Source: CAD feature listing. Evaluate the final solid. Frame: model axes, mm. Give positions to 0.01 mm unless a question says otherwise; leave off trailing zeros. Order: outer loops, then holes, each group sorted by start corner. A loop starts at its lowest first (then second) coordinate and runs counter-clockwise, first axis right, second up. Notation, with made-up numbers: M 81.5,69.25 L 93.5,69.25 A23 ccw 93.5,87.25 Z; hole C 80.25,47 d1. An arc over 180 degrees is marked long. Return JSON: item names as keys, results as strings.
Autodesk Inventor part; units mm, degrees
ref_plane "YZ Plane" through (0, 0, 0) normal (1, 0, 0) x (0, 1, 0)
ref_plane "XZ Plane" through (0, 0, 0) normal (0, 1, 0) x (-1, 0, 0)
ref_plane "XY Plane" through (0, 0, 0) normal (0, 0, 1) x (1, 0, 0)
sketch "Szkic1" plane through (0, 0, 0) normal (0, 0, 1) x (1, 0, 0)
  circle A0 centre (0, 0) radius 6.5
  circle A1 centre (0, 0) radius 2
  dimension "d0" = 13
  dimension "d1" = 4
extrude "Wyciągnięcie proste1" add sketch "Szkic1" along normal blind 5
chamfer "Faza1" distance 0.2 angle 45 4 edges at (-2, 0, 5) (-6.5, 0, 5) (-6.5, 0, 0) (-2, 0, 0)
sketch "Szkic2" plane through (0, 0, 5) normal (0, 0, 1) x (1, 0, 0)
  circle A0 centre (0, 0) radius 6.5
  circle A1 centre (0, 0) radius 2
  circle A2 centre (0, 0) radius 5.5
  circle A3 centre (0, 0) radius 3
  dimension "d7" = 1
  dimension "d8" = 1
extrude "Wyciągnięcie proste2" cut sketch "Szkic2" against normal blind 0.2 contours A2
sketch "Szkic3" plane through (0, 0, 0) normal (0, 0, -1) x (-1, 0, 0)
  circle A0 centre (0, 0) radius 5.5
  circle A1 centre (0, 0) radius 6.3
  circle A2 centre (0, 0) radius 2.2
  circle A3 centre (0, 0) radius 3
extrude "Wyciągnięcie proste3" cut sketch "Szkic3" against normal blind 0.2 contours A0
properties part number "COTS_GENERIC_Bearing_13x4x5"
1. First-contact query: pin 1 (3 mm diameter, centred on x = 0, y = 0, fed in from +Z). Flat tip, straight axial feed; report the tip coordinate or a pass-through.
Evaluation:
{"pin 1": "passes through"}
2. Draft query along Y for faces 1 (the face through (2.4, -2.4, 4.8)), 2 (the face through (-5.158, 3.955, 2.468)), 3 (the face through (-2.4, -2.4, 0.2)), 4 (the face through (0, -6, 5)). Return one class per face: pulls with the +Y half, pulls with the -Y half, needs draft (parallel to the pull), parting line crosses it, or undercut.
Evaluation:
{"face 1": "undercut", "face 2": "parting line crosses it", "face 3": "undercut", "face 4": "needs draft"}
3. Section query C-C (z = 1.2). Return loops of the section in (x, y).
Evaluation:
{"outline": "C 0,0 d13; hole C 0,0 d4"}
4. Ray query, probe 1 along Z at (x, y) = (3, -3); probe 2 along X at (y, z) = (0.75, 2.9); probe 3 along X at (y, z) = (-1, 3). Return the intervals inside material, ascending.
Evaluation:
{"probe 1": "z = 0.2 to 4.8", "probe 2": "x = -6.46 to -1.85, 1.85 to 6.46", "probe 3": "x = -6.42 to -1.73, 1.73 to 6.42"}
